For this review, take the finished solid that the model builds, in its own axes (mm). A direction names the side the tool comes from. Give positions to 0.01 mm unless a question says otherwise; leave off trailing zeros. Order: outer loops, then holes, each group sorted by start corner. A loop starts at its lowest first (then second) coordinate and runs counter-clockwise, first axis right, second up.
Item 1: Consider section B-B (x = -35). Give the boundary of the cut face in (y, z), plus the area to 3 significant figures.
Item 2: Machinability: for faces 5 (the cylindrical face through (-3.347, 7.266, 5.24)), 6 (the flat face through (7.793, 39.096, 0.986)), 7 (the flat face through (3.685, 19.998, 2.958)), which of the approach directions +Z, -Z, +X, -X, +Y, -Y give a long, thin tool a straight path to every point of the face, cutting with its end or side? Answer none if there is none.
Item 3: Consider section A-A (z = 3). Give the number of separate pieces and of enclosed holes in the cut face, plus the area to 3 significant figures.
Item 4: For P1, Ø3, axis at x = 12, y = 35, coming from the +Z side; P2, Ø2, axis at x = -6.5, z = 1.5, coming from the -Y side; P3, Ø2, axis at y = 23, z = 2, coming from the +X side; P4, Ø4, axis at x = 11.5, y = 34.5, coming from the -Z side, all flat-tipped, find the tip position at first contact; note any pin that passes through.
Item 5: The part is to be moulded in two halves that separate along Y. For faces 1 (the flat face through (-10.66, 17.23, 2.96)), 2 (the cylindrical face through (8.48, 2.08, 5.24)), 3 (the flat face through (-15.345, 30.525, 2.958)), 4 (the flat face through (-11, 19, 6)), say which applies: released by +Y, released by -Y, zero draft, split by the parting line, or undercut.
Item 6: For probe 1 along X at (y, z) = (23, 5.25); probe 2 along X at (y, z) = (26, 1.75); probe 3 along X at (y, z) = (27, 4), list the stretches that pass through material, from the lowest coordinate up.
Item 7: Consider section C-C (y = 35). Give the boundary of the cut face in (x, z), plus the area to 3 significant figures.
Item 8: Consider section D-D (x = 0). Give the boundary of the cut face in (y, z).
```python
from build123d import *

# Parameters (mm, degrees)
SKETCH1_R               = 3
SKETCH1_R_2             = 4
SKETCH1_R_3             = 2.5
BOSS_EXTRUDE1_DEPTH     = 6
CUT_EXTRUDE1_DEPTH      = 62.10646447
CUT_EXTRUDE1_DEPTH_BACK = 62.10646447
CUT_EXTRUDE2_START      = -2
SKETCH4_R               = 8
CUT_EXTRUDE2_DEPTH      = 2
FILLET1_START           = 4
FILLET1_DEPTH           = 2
FILLET2_R               = 0.5
CUT_EXTRUDE4_DEPTH      = 2


with BuildPart() as part:
    # Sketch1 → Boss-Extrude1 (new body)
    with BuildSketch(Plane.XY):
        with BuildLine():
            Line((19.567567568, 32.405405405), (7.567567568, -2.594594595))
            ThreePointArc((7.567567568, -2.594594595), (3.516422912, -7.185733776), (-2.594594595, -7.567567568))
            Line((-2.594594595, -7.567567568), (-37.594594595, 4.432432432))
            ThreePointArc((-37.594594595, 4.432432432), (-42.984429152, 11.50111011), (-38.516422912, 19.185733776))
            Line((-38.516422912, 19.185733776), (8.483577088, 42.185733776))
            ThreePointArc((8.483577088, 42.185733776), (17.293075573, 40.998612422), (19.567567568, 32.405405405))
        make_face()
        with Locations((-35, 12)):
            Circle(SKETCH1_R, mode=Mode.SUBTRACT)
        Circle(SKETCH1_R_2, mode=Mode.SUBTRACT)
        with Locations((12, 35)):
            Circle(SKETCH1_R_3, mode=Mode.SUBTRACT)
    extrude(amount=BOSS_EXTRUDE1_DEPTH)

    # Sketch2 → Cut-Extrude1 (cut, two sides: drawn at the far end of the back side and taken through both)
    with BuildSketch(Plane.XY.offset(6).offset(-CUT_EXTRUDE1_DEPTH_BACK)):
        with BuildLine():
            Line((-27.3724879, 17.959246424), (-15.522864255, 23.75799842))
            ThreePointArc((-15.522864255, 23.75799842), (-14.377048473, 23.829592256), (-13.516209876, 23.070002633))
            Line((-13.516209876, 23.070002633), (-7.71745788, 11.220378988))
            ThreePointArc((-7.71745788, 11.220378988), (-7.940043134, 9.568598022), (-9.551269449, 9.142130773))
            Line((-9.551269449, 9.142130773), (-27.199645091, 15.193002422))
            ThreePointArc((-27.199645091, 15.193002422), (-28.21023907, 16.518379486), (-27.3724879, 17.959246424))
        make_face()
        with BuildLine():
            Line((-25.513513514, 11.918918919), (-10.378378378, 6.72972973))
            ThreePointArc((-10.378378378, 6.72972973), (-8.513513514, 2.918918919), (-12.324324324, 1.054054054))
            Line((-12.324324324, 1.054054054), (-27.459459459, 6.243243243))
            ThreePointArc((-27.459459459, 6.243243243), (-29.324324324, 10.054054054), (-25.513513514, 11.918918919))
        make_face()
        with BuildLine():
            Line((-9.923342988, 24.828214089), (-4.124590991, 12.978590444))
            ThreePointArc((-4.124590991, 12.978590444), (-2.683724054, 12.140839274), (-1.358346989, 13.151433254))
            Line((-1.358346989, 13.151433254), (4.692524659, 30.799808895))
            ThreePointArc((4.692524659, 30.799808895), (4.26605741, 32.41103521), (2.614276444, 32.633620464))
            Line((2.614276444, 32.633620464), (-9.235347201, 26.834868468))
            ThreePointArc((-9.235347201, 26.834868468), (-9.994936824, 25.974029871), (-9.923342988, 24.828214089))
        make_face()
        with BuildLine():
            Line((6.243243243, 27.459459459), (1.054054054, 12.324324324))
            ThreePointArc((1.054054054, 12.324324324), (2.918918919, 8.513513514), (6.72972973, 10.378378378))
            Line((6.72972973, 10.378378378), (11.918918919, 25.513513514))
            ThreePointArc((11.918918919, 25.513513514), (10.054054054, 29.324324324), (6.243243243, 27.459459459))
        make_face()
    extrude(amount=CUT_EXTRUDE1_DEPTH + CUT_EXTRUDE1_DEPTH_BACK, mode=Mode.SUBTRACT)

    # Sketch4 → Cut-Extrude2 (cut)
    with BuildSketch(Plane.XY.offset(6).offset(CUT_EXTRUDE2_START)):
        Circle(SKETCH4_R)
    extrude(amount=CUT_EXTRUDE2_DEPTH, mode=Mode.SUBTRACT)

    # Fillet1: read off the stored shape, not the designer's step
    # Fillet1 outline → Fillet1 (cut)
    with BuildSketch(Plane.XY.offset(FILLET1_START)):
        with BuildLine():
            ThreePointArc((9.402223, 2.75648375), (8.465816464, 2.080853575), (7.516690715, 2.738496066))
            ThreePointArc((7.516690715, 2.738496066), (7.999635991, 0.076315279), (7.567567568, -2.594594595))
            Line((7.567567568, -2.594594595), (9.402223, 2.75648375))
        make_face()
        with BuildLine():
            ThreePointArc((-2.594594595, -7.567567568), (-4.968729766, -6.269906261), (-6.774532102, -4.255081057))
            ThreePointArc((-6.774532102, -4.255081057), (-6.837610332, -5.40805741), (-7.945672939, -5.732912135))
            Line((-7.945672939, -5.732912135), (-2.594594595, -7.567567568))
        make_face()
    extrude(amount=FILLET1_DEPTH, mode=Mode.SUBTRACT)

    # Fillet2
    fillet2_edges = [part.edges().sort_by_distance(p)[0] for p in [
        (-3.516422912, 7.185733776, 4),
        (8.465816464, 2.080853575, 4),
        (-6.837610332, -5.40805741, 4),
    ]]
    fillet(fillet2_edges, radius=FILLET2_R)

    # Sketch5 → Cut-Extrude4 (cut)
    with BuildSketch(Plane(origin=(0, 0, 0), x_dir=(-1, 0, 0), z_dir=(0, 0, -1))):
        with BuildLine():
            Line((-7.12054628, 36.091298034), (-8.483577088, 42.185733776))
            ThreePointArc((-8.483577088, 42.185733776), (-17.293075573, 40.998612422), (-19.567567568, 32.405405405))
            Line((-19.567567568, 32.405405405), (-13.690203108, 30.2943424))
            ThreePointArc((-13.690203108, 30.2943424), (-8.691827767, 31.250867237), (-7.12054628, 36.091298034))
        make_face()
    extrude(amount=-CUT_EXTRUDE4_DEPTH, mode=Mode.SUBTRACT)


solid = part.part
```
Resolved:
1. outline: (3.54, 0) - (9, 0) - (9, 6) - (3.54, 6) - close; (15, 0) - (20.91, 0) - (20.91, 6) - (15, 6) - close
1. area: 68.2 mm2
2. face 5: +Z
2. face 6: -Z, +X
2. face 7: +Z, -Z
3. separate pieces: 1
3. enclosed holes: 7
3. area: 1,230 mm2
4. P1: passes through
4. P2: stops at y = -6.57
4. P3: stops at x = 16.69
4. P4: stops at z = 2
5. face 1: undercut
5. face 2: released by -Y
5. face 3: released by +Y
5. face 4: zero draft
6. probe 1: x = -30.72 to -17.07, -13.48 to -9.03, 2.02 to 4.71, 11.06 to 16.34
6. probe 2: x = -24.59 to -9.99, 3.05 to 5.74, 12.04 to 17.37
6. probe 3: x = -22.55 to -8.9, 3.39 to 6.09, 12.04 to 17.71
7. outline: (-6.2, 0) - (7, 0) - (7, 2) - (9.5, 2) - (9.5, 6) - (-6.2, 6) - close; (14.5, 2) - (20, 2) - (20, 6) - (14.5, 6) - close
7. area: 111 mm2
8. outline: (-8, 0) - (-4, 0) - (-4, 4) - (-8, 4) - close; (4, 0) - (17.11, 0) - (17.11, 6) - (8, 6) - (8, 4.5) arc R0.5 cw to (7.5, 4) - (4, 4) - close; (31.35, 0) - (38.03, 0) - (38.03, 6) - (31.35, 6) - close
